Verification items for the finished model (mm, model axes). A direction names the side the tool comes from. Round coordinates to 2 decimals unless told otherwise and drop trailing zeros. Write each loop counter-clockwise with the first axis right and the second up, starting at its lowest first coordinate (ties: lowest second). Pieces come first, ordered by that corner, then holes. Notation, with made-up numbers: M -28.5,58.25 L -9.5,58.25 A7 ccw -9.5,62.25 Z; hole C 80,88.25 d2. An arc over 180 degrees is marked long. Write each question's results on one line, items separated by ' | '.
from build123d import *

# Parameters (mm, degrees)
F0_W         = 50.964426635
F0_H         = 1
F1_DEPTH     = 40
F2_DEPTH     = 45
F3_DEPTH     = 5
F4_START     = 1
F4_DEPTH     = 44.001
F6_START     = 1
F6_DEPTH     = 38
F7_START     = 1
F7_DEPTH     = 44.001
F9_DEPTH     = 25
F11_DEPTH    = 25
F12_T1_DEPTH = 1
F12_T3_DEPTH = 1


# Not quite as in the source:
# - a fillet or chamfer that OpenCascade refuses, or shapes differently, is made with other operations: its cross-section is extruded or revolved along the edge and cut away or added


with BuildPart() as f1:
    # F0 (on Front) → F1 (new body)
    with BuildSketch(Plane.XZ):
        Polygon((25.4822133175, 48.8744375096), (0, 90), (-25.4822133175, 48.8744375096), (-25.4822133175, 1), (25.4822133175, 1), align=None)
        with BuildLine():
            ThreePointArc((-16.8351454988, 38.3754507383), (-12.9010914993, 51.3524985976), (0, 47.1760898363))
            ThreePointArc((0, 47.1760898363), (12.8897582031, 51.3584134172), (16.847382477, 38.3979000332))
            ThreePointArc((16.847382477, 38.3979000332), (15.916282128, 37.1777103045), (14.6589247027, 36.2974471967))
            ThreePointArc((14.6589247027, 36.2974471967), (6.3677193864, 30.6369091459), (0, 22.8755995631))
            ThreePointArc((0, 22.8755995631), (-6.3946665322, 30.6177021843), (-14.6752906719, 36.297770574))
            ThreePointArc((-14.6752906719, 36.297770574), (-15.914547628, 37.1709794451), (-16.8351454988, 38.3754507383))
        make_face(mode=Mode.SUBTRACT)
        with BuildLine():
            Line((-2.5, 73.7544666829), (-2.5, 77.2864818573))
            ThreePointArc((-2.5, 77.2864818573), (0, 79.7864818573), (2.5, 77.2864818573))
            Line((2.5, 77.2864818573), (2.5, 73.7544666829))
            ThreePointArc((2.5, 73.7544666829), (0, 67.8049769402), (-2.5, 73.7544666829))
        make_face(mode=Mode.SUBTRACT)
        with BuildLine():
            ThreePointArc((16.847382477, 38.3979000332), (12.8897582031, 51.3584134172), (0, 47.1760898363))
            ThreePointArc((0, 47.1760898363), (-12.9010914993, 51.3524985976), (-16.8351454988, 38.3754507383))
            ThreePointArc((-16.8351454988, 38.3754507383), (-15.914547628, 37.1709794451), (-14.6752906719, 36.297770574))
            ThreePointArc((-14.6752906719, 36.297770574), (-6.3946665322, 30.6177021843), (0, 22.8755995631))
            ThreePointArc((0, 22.8755995631), (6.3677193864, 30.6369091459), (14.6589247027, 36.2974471967))
            ThreePointArc((14.6589247027, 36.2974471967), (15.916282128, 37.1777103045), (16.847382477, 38.3979000332))
        make_face()
        with BuildLine():
            ThreePointArc((2.5, 77.2864818573), (0, 79.7864818573), (-2.5, 77.2864818573))
            Line((-2.5, 77.2864818573), (-2.5, 73.7544666829))
            ThreePointArc((-2.5, 73.7544666829), (0, 67.8049769402), (2.5, 73.7544666829))
            Line((2.5, 73.7544666829), (2.5, 77.2864818573))
        make_face()
        with Locations((0, 0.5)):
            Rectangle(F0_W, F0_H)
        Polygon((-25.4822133175, 1), (-25.4822133175, 48.8744375096), (-26.4822133175, 47.2605446354), (-26.4822133175, 0), (-25.4822133175, 0), align=None)
        Polygon((26.4822133175, 47.2605446354), (25.4822133175, 48.8744375096), (25.4822133175, 1), (25.4822133175, 0), (26.4822133175, 0), align=None)
    extrude(amount=F1_DEPTH)

    # F0 (on Front) → F2 (join)
    with BuildSketch(Plane.XZ):
        Polygon((-26.4822133175, 47.2605446354), (-25.4822133175, 48.8744375096), (-25.4822133175, 50.7730291479), (-34.5699527606, 36.1063912187), (-37.6622251316, 38.0224244453), (-25.4822133175, 57.679658719), (0, 98.8052212095), (25.4822133175, 57.679658719), (37.6622251316, 38.0224244453), (34.5699527606, 36.1063912187), (25.4822133175, 50.7730291479), (25.4822133175, 48.8744375096), (26.4822133175, 47.2605446354), (34.2466115735, 34.7296376181), (39.0389787322, 37.6990832582), (0, 100.7038128478), (-39.0389787322, 37.6990832582), (-34.2466115735, 34.7296376181), align=None)
        Polygon((-25.4822133175, 48.8744375096), (0, 90), (25.4822133175, 48.8744375096), (25.4822133175, 50.7730291479), (25.4822133175, 57.679658719), (0, 98.8052212095), (-25.4822133175, 57.679658719), (-25.4822133175, 50.7730291479), align=None)
        Polygon((-34.5699527606, 36.1063912187), (-25.4822133175, 50.7730291479), (-25.4822133175, 57.679658719), (-37.6622251316, 38.0224244453), align=None)
        Polygon((25.4822133175, 57.679658719), (25.4822133175, 50.7730291479), (34.5699527606, 36.1063912187), (37.6622251316, 38.0224244453), align=None)
    extrude(amount=F2_DEPTH)

    # F0 (on Front) → F3 (cut)
    with BuildSketch(Plane.XZ):
        with BuildLine():
            ThreePointArc((2.5, 77.2864818573), (0, 79.7864818573), (-2.5, 77.2864818573))
            Line((-2.5, 77.2864818573), (-2.5, 73.7544666829))
            ThreePointArc((-2.5, 73.7544666829), (0, 67.8049769402), (2.5, 73.7544666829))
            Line((2.5, 73.7544666829), (2.5, 77.2864818573))
        make_face()
        with Locations((0, 0.5)):
            Rectangle(F0_W, F0_H)
    extrude(amount=F3_DEPTH, mode=Mode.SUBTRACT)

    # F0 (on Front) → F4 (cut)
    with BuildSketch(Plane.XZ.offset(F4_START)):
        with BuildLine():
            ThreePointArc((16.847382477, 38.3979000332), (12.8897582031, 51.3584134172), (0, 47.1760898363))
            ThreePointArc((0, 47.1760898363), (-12.9010914993, 51.3524985976), (-16.8351454988, 38.3754507383))
            ThreePointArc((-16.8351454988, 38.3754507383), (-15.914547628, 37.1709794451), (-14.6752906719, 36.297770574))
            ThreePointArc((-14.6752906719, 36.297770574), (-6.3946665322, 30.6177021843), (0, 22.8755995631))
            ThreePointArc((0, 22.8755995631), (6.3677193864, 30.6369091459), (14.6589247027, 36.2974471967))
            ThreePointArc((14.6589247027, 36.2974471967), (15.916282128, 37.1777103045), (16.847382477, 38.3979000332))
        make_face()
    extrude(amount=F4_DEPTH, mode=Mode.SUBTRACT)

    # F0 (on Front) → F6 (cut)
    with BuildSketch(Plane.XZ.offset(F6_START)):
        Polygon((25.4822133175, 48.8744375096), (0, 90), (-25.4822133175, 48.8744375096), (-25.4822133175, 1), (25.4822133175, 1), align=None)
        with BuildLine():
            ThreePointArc((-16.8351454988, 38.3754507383), (-12.9010914993, 51.3524985976), (0, 47.1760898363))
            ThreePointArc((0, 47.1760898363), (12.8897582031, 51.3584134172), (16.847382477, 38.3979000332))
            ThreePointArc((16.847382477, 38.3979000332), (15.916282128, 37.1777103045), (14.6589247027, 36.2974471967))
            ThreePointArc((14.6589247027, 36.2974471967), (6.3677193864, 30.6369091459), (0, 22.8755995631))
            ThreePointArc((0, 22.8755995631), (-6.3946665322, 30.6177021843), (-14.6752906719, 36.297770574))
            ThreePointArc((-14.6752906719, 36.297770574), (-15.914547628, 37.1709794451), (-16.8351454988, 38.3754507383))
        make_face(mode=Mode.SUBTRACT)
        with BuildLine():
            Line((-2.5, 73.7544666829), (-2.5, 77.2864818573))
            ThreePointArc((-2.5, 77.2864818573), (0, 79.7864818573), (2.5, 77.2864818573))
            Line((2.5, 77.2864818573), (2.5, 73.7544666829))
            ThreePointArc((2.5, 73.7544666829), (0, 67.8049769402), (-2.5, 73.7544666829))
        make_face(mode=Mode.SUBTRACT)
        Polygon((-25.4822133175, 48.8744375096), (0, 90), (25.4822133175, 48.8744375096), (25.4822133175, 50.7730291479), (25.4822133175, 57.679658719), (0, 98.8052212095), (-25.4822133175, 57.679658719), (-25.4822133175, 50.7730291479), align=None)
        with BuildLine():
            ThreePointArc((2.5, 77.2864818573), (0, 79.7864818573), (-2.5, 77.2864818573))
            Line((-2.5, 77.2864818573), (-2.5, 73.7544666829))
            ThreePointArc((-2.5, 73.7544666829), (0, 67.8049769402), (2.5, 73.7544666829))
            Line((2.5, 73.7544666829), (2.5, 77.2864818573))
        make_face()
        Polygon((-34.5699527606, 36.1063912187), (-25.4822133175, 50.7730291479), (-25.4822133175, 57.679658719), (-37.6622251316, 38.0224244453), align=None)
        Polygon((25.4822133175, 57.679658719), (25.4822133175, 50.7730291479), (34.5699527606, 36.1063912187), (37.6622251316, 38.0224244453), align=None)
        with Locations((0, 0.5)):
            Rectangle(F0_W, F0_H)
    extrude(amount=F6_DEPTH, mode=Mode.SUBTRACT)

    # F0 (on Front) → F7 (cut)
    with BuildSketch(Plane.XZ.offset(F7_START)):
        with Locations((0, 0.5)):
            Rectangle(F0_W, F0_H)
    extrude(amount=F7_DEPTH, mode=Mode.SUBTRACT)

    # F8 (on face) → F9 (cut)
    with BuildSketch(Plane(origin=(-26.4822133175, 0, 0), x_dir=(0, -1, 0), z_dir=(-1, 0, 0))):
        with BuildLine():
            Line((34.9282032303, 1), (5.0717967697, 1))
            ThreePointArc((5.0717967697, 1), (3.7777015442, 0.8296291314), (2.5717967697, 0.3301270189))
            Line((2.5717967697, 0.3301270189), (2, 0))
            Line((2, 0), (38, 0))
            Line((38, 0), (37.4282032303, 0.3301270189))
            ThreePointArc((37.4282032303, 0.3301270189), (36.2222984558, 0.8296291314), (34.9282032303, 1))
        make_face()
    extrude(amount=-F9_DEPTH, mode=Mode.SUBTRACT)

    # F10 (on face) → F11 (cut)
    with BuildSketch(Plane.YZ.offset(26.4822133175)):
        with BuildLine():
            Line((-37.4282032303, 0.3301270189), (-38, 0))
            Line((-38, 0), (-2, 0))
            Line((-2, 0), (-2.5717967697, 0.3301270189))
            ThreePointArc((-2.5717967697, 0.3301270189), (-3.7777015442, 0.8296291314), (-5.0717967697, 1))
            Line((-5.0717967697, 1), (-34.9282032303, 1))
            ThreePointArc((-34.9282032303, 1), (-36.2222984558, 0.8296291314), (-37.4282032303, 0.3301270189))
        make_face()
    extrude(amount=-F11_DEPTH, mode=Mode.SUBTRACT)

    # F12: fillet of radius 5 on 4 edges, made by hand

    # F12_s2 → F12_t1 (join)
    with BuildSketch(Plane.XZ):
        with BuildLine():
            ThreePointArc((25.4822133175, 0), (24.0633521476, 0.7434164903), (22.4822133175, 1))
            Line((22.4822133175, 1), (25.4822133175, 1))
            Line((25.4822133175, 1), (25.4822133175, 0))
        make_face()
        with BuildLine():
            ThreePointArc((-22.4822133175, 1), (-24.0633521476, 0.7434164903), (-25.4822133175, 0))
            Line((-25.4822133175, 0), (-25.4822133175, 1))
            Line((-25.4822133175, 1), (-22.4822133175, 1))
        make_face()
    extrude(amount=F12_T1_DEPTH)

    # F12_s4 → F12_t3 (join)
    with BuildSketch(Plane.XZ.offset(39)):
        with BuildLine():
            ThreePointArc((25.4822133175, 0), (24.0633521476, 0.7434164903), (22.4822133175, 1))
            Line((22.4822133175, 1), (25.4822133175, 1))
            Line((25.4822133175, 1), (25.4822133175, 0))
        make_face()
        with BuildLine():
            ThreePointArc((-25.4822133175, 0), (-24.0633521476, 0.7434164903), (-22.4822133175, 1))
            Line((-22.4822133175, 1), (-25.4822133175, 1))
            Line((-25.4822133175, 1), (-25.4822133175, 0))
        make_face()
    extrude(amount=F12_T3_DEPTH)


solid = f1.part
1) Sectioned sample at D-D, the plane z = 92. Record the cut outline in (x, y).
Calculated:
outline: M -5.39,-45 L 5.39,-45 L 5.39,0 L -5.39,0 Z; hole M -4.22,-39 L 4.22,-39 L 4.22,-1 L -4.22,-1 Z
2) Access from +Z, -Z, +X, -X, +Y, -Y to the whole of each face (thin tool, end or side, straight path). Record for faces 4 (the flat face through (-36.14, -19.73, 37.08)), 5 (the flat face through (25.482, -20, 25)), 6 (the flat face through (-26.482, -20, 24)).
Calculated:
face 4: none | face 5: -Z | face 6: -Z, +Y, -Y
3) Sectioned sample at C-C, the plane y = -11.5. Record the cut outline in (x, z), and give its area (3 significant figures).
Calculated:
outline: M -39.04,37.7 L -34.25,34.73 L -26.48,47.26 L -26.48,1 L -25.48,1 L -25.48,50.77 L -34.57,36.11 L -37.66,38.02 L 0,98.81 L 37.66,38.02 L 34.57,36.11 L 25.48,50.77 L 25.48,1 L 26.48,1 L 26.48,47.26 L 34.25,34.73 L 39.04,37.7 L 0,100.7 Z | area: 283 mm²
4) Sectioned sample at A-A, the plane z = 40. Record the cut outline in (x, y), and give its area (3 significant figures).
Calculated:
outline: M -37.61,-45 L -30.98,-45 L -30.98,0 L -37.61,0 Z; M -26.48,-40 L -17.54,-40 L -17.54,-39 L -25.48,-39 L -25.48,-1 L 25.48,-1 L 25.48,-39 L 17.54,-39 L 17.54,-40 L 26.48,-40 L 26.48,0 L -26.48,0 Z; M 30.98,-45 L 37.61,-45 L 37.61,0 L 30.98,0 Z; hole M -36.44,-39 L -32.16,-39 L -32.16,-1 L -36.44,-1 Z; hole M 32.16,-39 L 36.44,-39 L 36.44,-1 L 32.16,-1 Z | area: 419 mm²
5) Material ranges on line 1 (Y direction, x = -24.5, z = 18.5); line 2 (X direction, y = -2, z = 17.5); line 3 (X direction, y = -29, z = 78), recorded low to high. Write a range as [from, to].
Calculated:
line 1: y = [-40, -39], [-1, 0] | line 2: x = [-26.48, -25.48], [25.48, 26.48] | line 3: x = [-14.07, -12.89], [12.89, 14.07]
6) Draft check along X on faces 1 (the flat face through (19.793, -22.185, 68.76)), 2 (the flat face through (-19.25, -22.18, 69.64)), 3 (the flat face through (6, -40, 26)). Enter one of: pulls with the +X half, pulls with the -X half, needs draft (parallel to the pull), parting line crosses it, or undercut.
Calculated:
face 1: pulls with the +X half | face 2: pulls with the -X half | face 3: undercut
7) Sectioned sample at B-B, the plane x = 9. Record the cut outline in (y, z), and give its area (3 significant figures).
Calculated:
outline: M -45,75.47 L -40,75.47 L -40,52.42 L -39,52.42 L -39,84.28 L -1,84.28 L -1,1 L 0,1 L 0,86.18 L -45,86.18 Z; M -40,1 L -39,1 L -39,32.82 L -40,32.82 Z | area: 276 mm²
8) Depth check by flat-ended pin: P1, Ø6.5, axis at x = 0, z = 71.3, coming from the +Y side; P2, Ø1, axis at x = -5, z = 29.5, coming from the -Y side; P3, Ø4, axis at y = -32.5, z = 87, coming from the -X side. Enter the tip coordinate at first touch or a pass-through.
Calculated:
P1: stops at y = -39 | P2: stops at y = -40 | P3: stops at x = -9.73
